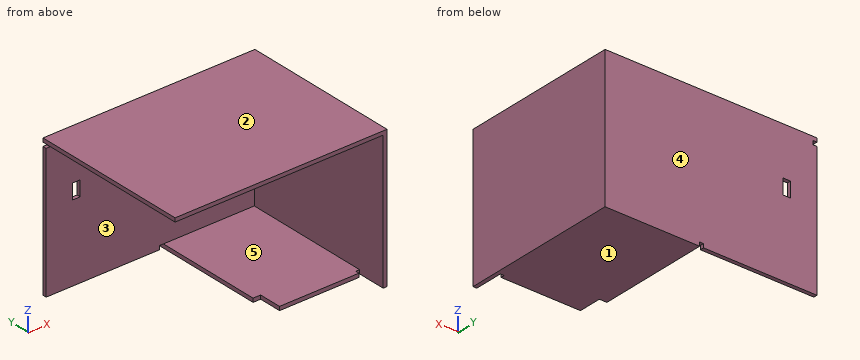
Autodesk Inventor part; units mm, degrees
ref_plane "YZ Plane" through (0, 0, 0) normal (1, 0, 0) x (0, 1, 0)
ref_plane "XZ Plane" through (0, 0, 0) normal (0, 1, 0) x (-1, 0, 0)
ref_plane "XY Plane" through (0, 0, 0) normal (0, 0, 1) x (1, 0, 0)
sketch "Sketch1" plane through (0, 0, 0) normal (0, 1, 0) x (-1, 0, 0)
  line L0 (58, 35) -> (-50, 35)
  line L1 (-50, 35) -> (-50, -35)
  line L2 (-50, -35) -> (58, -35)
  line L3 (58, -35) -> (58, 35)
  point P0 (0, 0)
  dimension "d1" = 70
  dimension "d36" = 50
  dimension "d37" = 58
  dimension "d38" = 35
extrude "Extrusion1" add sketch "Sketch1" against normal blind 2
sketch "Sketch2" plane through (0, 0, 0) normal (0, 1, 0) x (-1, 0, 0)
  line L0 (-50, 35) -> (58, 35)
  line L1 (58, 35) -> (-50, 35)
  line L2 (-50, 35) -> (-50, 37)
  line L3 (-50, 37) -> (58, 37)
  line L4 (58, 37) -> (58, 35)
  point P0 (0, 0)
  dimension "d4" = 2
extrude "Extrusion2" add sketch "Sketch2" against normal blind 84
sketch "Sketch3" plane through (0, 0, 0) normal (0, 1, 0) x (-1, 0, 0)
  line L0 (58, -35) -> (-50, -35)
  line L1 (-50, -35) -> (-52, -35)
  line L2 (-52, -35) -> (-52, 37)
  line L3 (-52, 37) -> (-50, 37)
  line L4 (-50, 37) -> (-50, -35)
  point P0 (0, 0)
  dimension "d7" = 2
extrude "Extrusion3" add sketch "Sketch3" against normal blind 84
sketch "Sketch4" plane through (0, 0, 0) normal (0, 1, 0) x (-1, 0, 0)
  line L0 (-50, -35) -> (-52, -35)
  line L1 (-52, -35) -> (-2, -35)
  line L2 (-2, -35) -> (-2, -37)
  line L3 (-2, -37) -> (-52, -37)
  line L4 (-52, -37) -> (-52, -35)
  point P0 (0, 0)
  dimension "d10" = 50
  dimension "d11" = 2
extrude "Extrusion4" add sketch "Sketch4" against normal blind 71
sketch "Sketch5" plane through (52, 0, -37) normal (0, 0, -1) x (-1, 0, 0)
  line L0 (50, -2) -> (50, -71)
  line L1 (50, -71) -> (46, -71)
  line L2 (46, -71) -> (46, -59)
  line L3 (46, -59) -> (50, -59)
  line L4 (50, -59) -> (50, -71)
  point P0 (52, 0)
  dimension "d14" = 4
  dimension "d15" = 12
extrude "Extrusion5" cut sketch "Sketch5" against normal blind 3
sketch "Sketch6" plane through (0, 0, 0) normal (0, 1, 0) x (-1, 0, 0)
  line L0 (58, -35) -> (58, 37)
  line L1 (58, 37) -> (60, 37)
  line L2 (60, 37) -> (60, -37)
  line L3 (-2, -37) -> (-2, -35)
  line L4 (60, -37) -> (-2, -37)
  line L5 (58, -35) -> (-2, -35)
  line L6 (-2, -37) -> (-2, -35)
  point P0 (0, 0)
  dimension "d18" = 2
extrude "Extrusion6" add sketch "Sketch6" against normal blind 2
sketch "Sketch7" plane through (0, -2, 0) normal (0, -1, 0) x (1, 0, 0)
  line L0 (2, -35) -> (2, -37)
  line L1 (2, -37) -> (0, -37)
  line L2 (0, -37) -> (0, -35)
  line L3 (0, -35) -> (2, -35)
  line L4 (2, -35) -> (2, -37)
  line L5 (2, -37) -> (2, -35)
  point P0 (0, 0)
  point P1 (1, -37)
  point P2 (1, -35)
  point P3 (2, -36)
  point P4 (0, -36)
  dimension "d21" = 2
  dimension "d22" = 2
sketch "Sketch8" plane through (0, -2, 0) normal (0, -1, 0) x (1, 0, 0)
  line L0 (50, 35) -> (-58, 35)
  line L1 (-60, 37) -> (-60, -37)
  line L2 (-58, 35) -> (-60, 35)
  line L3 (-60, 35) -> (-60, 37)
  line L4 (-60, 37) -> (-58, 37)
  line L5 (-58, 37) -> (-58, 35)
  point P0 (0, 0)
extrude "Extrusion7" add sketch "Sketch8" along normal blind 82
sketch "Sketch9" plane through (0, -2, 0) normal (0, -1, 0) x (1, 0, 0)
  line L0 (-60, 37) -> (-60, 35)
  line L1 (-60, 35) -> (-58, 35)
  line L2 (-58, 35) -> (-58, 33)
  line L3 (-58, 33) -> (-60, 33)
  line L4 (-60, 33) -> (-60, 35)
  point P0 (0, 0)
  dimension "d25" = 2
  dimension "d26" = 2
extrude "Extrusion8" cut sketch "Sketch9" against normal blind 2
extrude "Extrusion9" cut sketch "Sketch7" against normal blind 2
sketch "Sketch10" plane through (0, -71, 0) normal (0, -1, 0) x (1, 0, 0)
  line L0 (52, 37) -> (52, -37)
  line L1 (2, -35) -> (50, -35)
  line L2 (52, -37) -> (50, -37)
  line L3 (50, -37) -> (50, -35)
  line L4 (50, -35) -> (52, -35)
  line L5 (52, -35) -> (52, -37)
  point P0 (0, 0)
extrude "Extrusion10" add sketch "Sketch10" along normal blind 13
sketch "Sketch11" plane through (0, -71, 0) normal (0, -1, 0) x (1, 0, 0)
  line L0 (50, 35) -> (50, -37)
  line L1 (50, -35) -> (6, -35)
  line L2 (50, -37) -> (48, -37)
  line L3 (48, -37) -> (48, -35)
  line L4 (48, -35) -> (50, -35)
  line L5 (50, -35) -> (50, -37)
  point P0 (0, 0)
  dimension "d33" = 2
extrude "Extrusion11" cut sketch "Sketch11" against normal blind 2
sketch "Sketch12" plane through (0, 0, 0) normal (0, 1, 0) x (1, 0, 0)
  line L0 (-42, -3.5) -> (-46, -3.5)
  line L1 (-46, -3.5) -> (-46, -11.5)
  line L2 (-46, -11.5) -> (-42, -11.5)
  line L3 (-42, -11.5) -> (-42, -3.5)
  line L4 (-42, -3.5) -> (-46, -11.5) construction
  line L5 (-46, -3.5) -> (-42, -11.5) construction
  line L6 (0, 37) -> (-60, 37)
  line L7 (-60, 37) -> (-60, -33)
  point P0 (0, 0)
  point P1 (-44, -7.5)
  dimension "d39" = 44.5
  dimension "d41" = 4
  dimension "d42" = 8
  dimension "d43" = 14
extrude "Extrusion12" cut sketch "Sketch12" against normal blind 10
properties part number "lid_3DPrint"
Design review of the part built by this model. Coordinates are the model's own, in mm. Face numbers are marked on the shaded views. A direction names the side the tool comes from. Give positions to 0.01 mm unless a question says otherwise; leave off trailing zeros. Loops run counter-clockwise (first coordinate to the right, second up) from the corner with the lowest first, then second, coordinate; pieces in that order, holes last. Notation, with made-up numbers: M 74.5,-37.75 L 78.5,-37.75 A21 ccw 78.5,-4.75 Z; hole C -25,78 d10. An arc over 180 degrees is marked long. Write item = value, one per line.
Q1. We need section A-A (y = -67.5). Give the boundary of the cut face in (x, z), plus the area to 3 significant figures.
Output values:
outline = M -60,35 L 50,35 L 50,-35 L 6,-35 L 6,-37 L 52,-37 L 52,37 L -60,37 Z
area = 456 mm^2
Q2. We need section D-D (y = -13.5). Give the boundary of the cut face in (x, z), plus the area to 3 significant figures.
Output values:
outline = M -60,35 L 50,35 L 50,-35 L 2,-35 L 2,-37 L 52,-37 L 52,37 L -60,37 Z
area = 464 mm^2
Q3. We need section B-B (x = -38.5). Give the boundary of the cut face in (y, z), plus the area to 3 significant figures.
Output values:
outline = M -84,35 L -2,35 L -2,-37 L 0,-37 L 0,37 L -84,37 Z
area = 312 mm^2
Q4. To check wall thickness, follow line 1 (Z direction, x = 4.5, y = -58); line 2 (X direction, y = -10, z = 7); line 3 (Z direction, x = -2.5, y = -24). State the ranges of each line that lie inside material, in increasing order. Write a range as [from, to].
Output values:
line_1 = [-37, -35], [35, 37]
line_2 = [50, 52]
line_3 = [35, 37]
Q5. We need section C-C (z = -15.5). Give the boundary of the cut face in (x, y).
Output values:
outline = M -60,-2 L 50,-2 L 50,-84 L 52,-84 L 52,0 L -60,0 Z
Q6. Draft analysis for pull direction Z (two halves, no side actions). For the marked faces 1, 2 and 3, state which applies: +Z half, -Z half, draft (parallel to the pull), parting line (faces both ways), or undercut.
Output values:
face_1 = -Z half
face_2 = +Z half
face_3 = undercut
Q7. For the marked faces 4 and 5, list the 3-axis set-ups (+Z, -Z, +X, -X, +Y, -Y) from which the entire face can be reached by the end or side of a thin tool; tool diameter is ignored.
Output values:
face_4 = +Z, -Z, +X, -X, +Y
face_5 = -X, -Y
Q8. Insertion check: pin 1 (12 mm diameter, centred on x = -9.5, y = -36, fed in from -Z); pin 2 (10 mm diameter, centred on y = -75, z = -5, fed in from -X); pin 3 (0.6 mm diameter, centred on x = 1, y = -1, fed in from -Z). Each pin has a flat end and moves straight along its axis. Give the tip position at first contact, or say it passes through.
Output values:
pin_1 = 35
pin_2 = 50
pin_3 = -35
